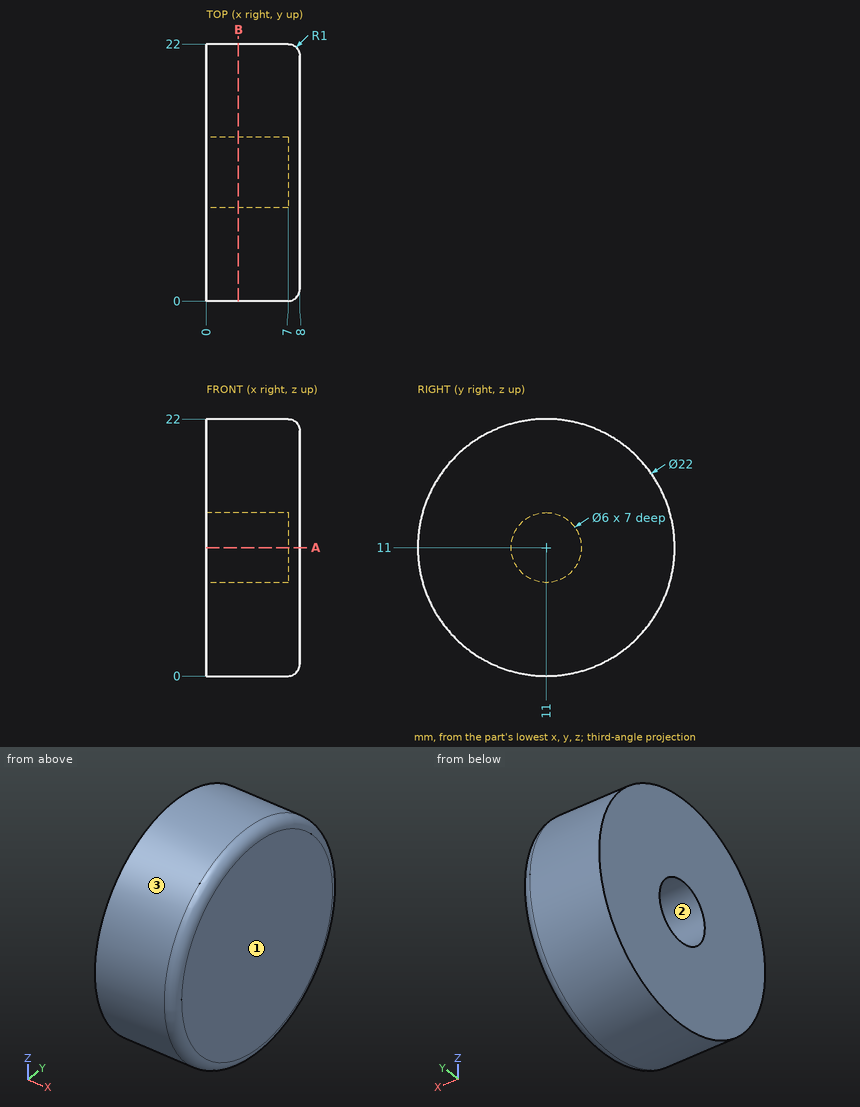
Geometry check sheet. Reference: drawing and pictorial views, mm from the part's lowest x, y, z. Coordinates: 2 decimals unless noted, no trailing zeros. Write each loop counter-clockwise with the first axis right and the second up, starting at its lowest first coordinate (ties: lowest second). Pieces come first, ordered by that corner, then holes. Notation, with made-up numbers: (22, 54) - (54, 54) arc R17 ccw to (54, 86) - close; hole circle Ø6 at (6.5, 41). An arc over 180 degrees is marked (long way). One line per question, with ' | ' between items. Start each with the question number.
1. Section check B-B (x = 2.75). Enter the section's corners in (y, z), plus the area to 3 significant figures.
2. Material ranges on line 1 along Y through (x, z) = (3.25, 11); line 2 along Y through (x, z) = (4.75, 9.25); line 3 along Z through (x, y) = (5.5, 11.5), recorded low to high.
3. Gauge pin test, flat ends, axial feed: P1, Ø2, axis at x = 2.5, y = 6.5, coming from the +Z side; P2, Ø1.8, axis at y = 12.5, z = 12, coming from the -X side; P3, Ø4, axis at x = 2, z = 19.5, coming from the -Y side. Record the tip position at first contact, or that the pin passes through.
4. Section check A-A (z = 11). Enter the section's corners in (x, y).
5. Draft check along Z on the marked faces 1, 2 and 3. Enter one of: released by +Z, released by -Z, zero draft, split by the parting line, or undercut.
Computed values:
1) outline: circle Ø22 at (11, 11); hole circle Ø6 at (11, 11) | area: 352 mm²
2) line 1: 0 to 8, 14 to 22 | line 2: 0.14 to 8.56, 13.44 to 21.86 | line 3: 0.01 to 8.04, 13.96 to 21.99
3) P1: z = 21.43 | P2: x = 7 | P3: y = 2.13
4) outline: (0, 0) - (7, 0) arc R1 ccw to (8, 1) - (8, 21) arc R1 ccw to (7, 22) - (0, 22) - (0, 14) - (7, 14) - (7, 8) - (0, 8) - close
5) face 1: zero draft | face 2: undercut | face 3: split by the parting line
